Part model, mm, in its own coordinate system. A direction names the side the tool comes from. Coordinates: 2 decimals unless noted, no trailing zeros. Loops run counter-clockwise (first coordinate to the right, second up) from the corner with the lowest first, then second, coordinate; pieces in that order, holes last. Notation, with made-up numbers: M 39,68.5 L 73,68.5 A34 ccw 73,102.5 Z; hole C 5,-4.75 d9. An arc over 180 degrees is marked long. Use a Markdown table: item, result. Add a question column.
1) Pull direction Z, two halves, no side cores. Call faces 3 (the flat face through (15, -19, -41)), 4 (the cylindrical face through (14.084, -25.296, 16.128)), 5 (the cylindrical face through (11.451, 39.923, 20.765)), 6 (the cylindrical face through (7.6, -15.02, 47.69)): released by +Z, released by -Z, zero draft, split by the parting line, or undercut.
2) Band-saw the part on A-A (y = 0). List the corners of the cut face in (x, z).
3) Tool access for faces 1 (the flat face through (0, 10.4, 0.7)), 2 (the flat face through (5, 22, -25)): list every direction of +Z, -Z, +X, -X, +Y, -Y with a clear straight run to the whole face (end or side of a thin tool).
4) Pin check, flat tips, straight feed: pin 1 Ø2 at (x, y) = (12.5, -21) entering from +Z; pin 2 Ø8 at (x, y) = (8, -39) entering from -Z; pin 3 Ø6 at (x, z) = (16, -26.5) entering from -Y; pin 4 Ø12 at (y, z) = (0, 0) entering from +X. Stop position of each tip, or through.
5) Band-saw the part on C-C (x = 11.75). List the corners of the cut face in (y, z), plus the area to 3 significant figures.
6) Wall check: probe 1 along Y at (x, z) = (10.5, 0); probe 2 along Y at (x, z) = (3.75, 0); probe 3 along Y at (x, z) = (13.5, 12). Give the ranges that are in metal, low to high. Write a range as from..to.
from build123d import *


with BuildPart() as part:
    # Croquis1 → Revolución1 (revolve)
    with BuildSketch(Plane.XY, mode=Mode.PRIVATE) as revoluci_n1_sk:
        with BuildLine():
            Line((0, 10), (0, 50))
            Line((0, 50), (15, 50))
            Line((15, 50), (15, 45))
            Line((15, 45), (8, 45))
            ThreePointArc((8, 45), (5.878679656, 44.121320344), (5, 42))
            Line((5, 42), (5, 33))
            ThreePointArc((5, 33), (5.878679656, 30.878679656), (8, 30))
            Line((8, 30), (20, 30))
            Line((20, 30), (20, 20))
            Line((20, 20), (10, 20))
            Line((10, 20), (10, 10))
            Line((10, 10), (0, 10))
        make_face()
    revolve(revoluci_n1_sk.sketch.rotate(Axis((-16.484758047, 0, 0), (1, 0, 0)), 90), axis=Axis((-16.484758047, 0, 0), (1, 0, 0)))


solid = part.part
Entries:
| question | item | result |
|---|---|---|
| 1 | face 3 | zero draft |
| 1 | face 4 | undercut |
| 1 | face 5 | undercut |
| 1 | face 6 | split by the parting line |
| 2 | outline | M 0,-50 L 15,-50 L 15,-45 L 8,-45 A3 cw 5,-42 L 5,-33 A3 cw 8,-30 L 20,-30 L 20,-20 L 10,-20 L 10,-10 L 0,-10 Z; M 0,10 L 10,10 L 10,20 L 20,20 L 20,30 L 8,30 A3 cw 5,33 L 5,42 A3 cw 8,45 L 15,45 L 15,50 L 0,50 Z |
| 3 | face 1 | +Z, -Z, -X, +Y, -Y |
| 3 | face 2 | +X |
| 4 | pin 1 | z = 45.83 |
| 4 | pin 2 | z = -35.71 |
| 4 | pin 3 | y = -44.04 |
| 4 | pin 4 | through |
| 5 | outline | C 0,0 d100; C 0,0 d60; hole C 0,0 d90; hole C 0,0 d40 |
| 5 | area | 3,060 mm2 |
| 6 | probe 1 | -50..-45, -30..-20, 20..30, 45..50 |
| 6 | probe 2 | -50..-10, 10..50 |
| 6 | probe 3 | -48.54..-43.37, -27.5..-16, 16..27.5, 43.37..48.54 |
